```python
from build123d import *

# Parameters (mm, degrees)
SKETCH_1_W       = 300
SKETCH_1_H       = 180
EXTRUDE_1_DEPTH  = 25
FILLET_1_R       = 10
F_20_0MM_1_D     = 20
F_20_0MM_1_DEPTH = 59
F_20_0MM_1_TIP   = 6.00860619
F_20_0MM_2_D     = 20
F_20_0MM_2_DEPTH = 59
F_20_0MM_2_TIP   = 6.00860619
CHAMFER_1_SIZE   = 2


with BuildPart() as part:
    # 草圖1 → 填料-伸長1 (new body)
    with BuildSketch(Plane.XY):
        with Locations((150, 90)):
            Rectangle(SKETCH_1_W, SKETCH_1_H)
    extrude(amount=EXTRUDE_1_DEPTH)

    # 圓角1
    fillet_1_edges = [part.edges().sort_by_distance(p)[0] for p in [
        (0, 180, 12.5),
        (300, 180, 12.5),
        (300, 0, 12.5),
        (0, 0, 12.5),
    ]]
    fillet(fillet_1_edges, radius=FILLET_1_R)

    # Ø20.0mm 定位孔1
    with Locations(Plane(origin=(25, 25, 25), x_dir=(1, 0, 0), z_dir=(0, 0, 1))):
        with Locations((0, 0), (0, 130), (125, 130), (250, 0), (250, 130)):
            Hole(F_20_0MM_1_D / 2, depth=F_20_0MM_1_DEPTH)
            with Locations((0, 0, -(F_20_0MM_1_DEPTH + F_20_0MM_1_TIP / 2))):  # 118° drill point
                Cone(0, F_20_0MM_1_D / 2, F_20_0MM_1_TIP, mode=Mode.SUBTRACT)

    # Ø20.0mm 定位孔2
    with Locations(Plane(origin=(150, 25, 25), x_dir=(1, 0, 0), z_dir=(0, 0, 1))):
        with Locations((0, 0)):
            Hole(F_20_0MM_2_D / 2, depth=F_20_0MM_2_DEPTH)
            with Locations((0, 0, -(F_20_0MM_2_DEPTH + F_20_0MM_2_TIP / 2))):  # 118° drill point
                Cone(0, F_20_0MM_2_D / 2, F_20_0MM_2_TIP, mode=Mode.SUBTRACT)

    # 導角1
    chamfer_1_edges = [part.edges().sort_by_distance(p)[0] for p in [
        (285, 155, 0),
        (285, 155, 25),
        (285, 25, 0),
        (285, 25, 25),
        (160, 155, 0),
        (160, 155, 25),
        (35, 155, 0),
        (35, 155, 25),
        (35, 25, 0),
        (35, 25, 25),
        (160, 25, 0),
        (160, 25, 25),
    ]]
    chamfer(chamfer_1_edges, length=CHAMFER_1_SIZE)


solid = part.part
```
For this review, take the finished solid that the model builds, in its own axes (mm). Round coordinates to 2 decimals unless told otherwise and drop trailing zeros. Write each loop counter-clockwise with the first axis right and the second up, starting at its lowest first coordinate (ties: lowest second). Pieces come first, ordered by that corner, then holes. Notation, with made-up numbers: (9, 56.5) - (68, 56.5) arc R15 ccw to (68, 76.5) - close; hole circle Ø4 at (7.25, -7). An arc over 180 degrees is marked (long way). Put each result on its own line as item: value.
Q1. Mouldability with a two-part tool opening along Y and no side actions: class faces 1 (the face through (148, 91, 0)), 2 (the face through (297.15, 176.99, 12.68)), 3 (the face through (15.46, 28, 12.35)), 4 (the face through (140.763, 21.17, 12.353)) as released by +Y, released by -Y, zero draft, split by the parting line, or undercut.
Solved:
face 1: zero draft
face 2: released by +Y
face 3: undercut
face 4: undercut
Q2. We need section B-B (x = 25). Give the boundary of the cut face in (y, z).
Solved:
outline: (0, 0) - (13, 0) - (15, 2) - (15, 23) - (13, 25) - (0, 25) - close; (35, 2) - (37, 0) - (143, 0) - (145, 2) - (145, 23) - (143, 25) - (37, 25) - (35, 23) - close; (165, 2) - (167, 0) - (180, 0) - (180, 25) - (167, 25) - (165, 23) - close
Q3. We need section D-D (x = 273). Count the separate pieces of the cut face and the enclosed holes in it, and give its area (3 significant figures).
Solved:
separate pieces: 3
enclosed holes: 0
area: 3,500 mm2
Q4. We need section C-C (z = 6.5). Give the boundary of the cut face in (x, y), and give its area (3 significant figures).
Solved:
outline: (0, 10) arc R10 ccw to (10, 0) - (290, 0) arc R10 ccw to (300, 10) - (300, 170) arc R10 ccw to (290, 180) - (10, 180) arc R10 ccw to (0, 170) - close; hole circle Ø20 at (25, 25); hole circle Ø20 at (25, 155); hole circle Ø20 at (150, 25); hole circle Ø20 at (150, 155); hole circle Ø20 at (275, 25); hole circle Ø20 at (275, 155)
area: 52,000 mm2
Q5. Wall thickness on probe 1 along Y at (x, z) = (275, 18.25); probe 2 along X at (y, z) = (16, 2.5); probe 3 along X at (y, z) = (149, 8): over which ranges is each line inside the solid? List them lowest first.
Solved:
probe 1: y = 0 to 15, 35 to 145, 165 to 180
probe 2: x = 0 to 20.64, 29.36 to 145.64, 154.36 to 270.64, 279.36 to 300
probe 3: x = 0 to 17, 33 to 142, 158 to 267, 283 to 300
Q6. We need section A-A (y = 25). Give the boundary of the cut face in (x, z).
Solved:
outline: (0, 0) - (13, 0) - (15, 2) - (15, 23) - (13, 25) - (0, 25) - close; (35, 2) - (37, 0) - (138, 0) - (140, 2) - (140, 23) - (138, 25) - (37, 25) - (35, 23) - close; (160, 2) - (162, 0) - (263, 0) - (265, 2) - (265, 23) - (263, 25) - (162, 25) - (160, 23) - close; (285, 2) - (287, 0) - (300, 0) - (300, 25) - (287, 25) - (285, 23) - close
Q7. Insertion check: pin 1 Ø16 at (x, y) = (25, 155) entering from -Z. The pin has a flat end and moves straight along its axis. Give the tip position at first contact, or say it passes through.
Solved:
pin 1: passes through
